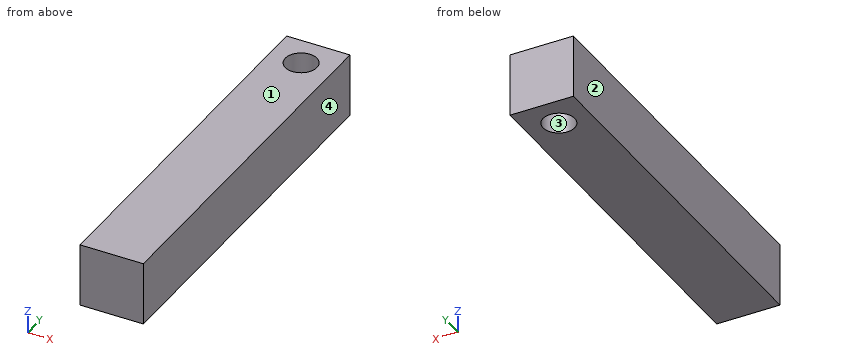
Autodesk Inventor part; units mm, degrees
ref_plane "YZ Plane" through (0, 0, 0) normal (1, 0, 0) x (0, 1, 0)
ref_plane "XZ Plane" through (0, 0, 0) normal (0, 1, 0) x (-1, 0, 0)
ref_plane "XY Plane" through (0, 0, 0) normal (0, 0, 1) x (1, 0, 0)
sketch "Sketch1" plane through (0, 0, 0) normal (0, 1, 0) x (-1, 0, 0)
  line L0 (0, 0) -> (-25.4, 0)
  line L1 (-25.4, 0) -> (-25.4, -25.4)
  line L2 (-25.4, -25.4) -> (0, -25.4)
  line L3 (0, -25.4) -> (0, 0)
  dimension "d0" = 25.4
  dimension "d1" = 25.4
extrude "Extrusion1" add sketch "Sketch1" along normal blind 152.4
sketch "Sketch2" plane through (25.4, 0, -25.4) normal (0, 0, -1) x (-1, 0, 0)
  circle A0 centre (12.7, 139.7) radius 6.35
  line L0 (0, 0) -> (0, 152.4)
  line L1 (0, 152.4) -> (25.4, 152.4)
  point P0 (25.4, 0)
  dimension "d4" = 12.7
  dimension "d5" = 12.7
  dimension "d6" = 12.7
extrude "Extrusion2" cut sketch "Sketch2" against normal blind 152.4
properties material "Aluminum 6061"
Can you work these out from the model? Positions are in its coordinate system, mm. Face numbers are marked on the shaded views. Give positions to 0.01 mm unless a question says otherwise; leave off trailing zeros. Loops run counter-clockwise (first coordinate to the right, second up) from the corner with the lowest first, then second, coordinate; pieces in that order, holes last. Notation, with made-up numbers: M 25.25,21.5 L 30.25,21.5 A12 cw 30.25,32.5 Z; hole C 18.5,86 d2. An arc over 180 degrees is marked long. Use one line per item in the form item = value. Start each with the question number.
(1) Thinking about a two-plate mould opening in X: for the marked faces 1, 2, 3 and 4, which applies, released by +X, released by -X, zero draft, split by the parting line, or undercut?
(2) I want a section at B-B, the plane y = 139.7. Write out the boundary of the cut face in (x, z), and give its area (3 significant figures).
(3) Please list where these lines run through material, in increasing order: line 1 (Y direction, x = 12.75, z = -14); line 2 (Y direction, x = 17.25, z = -15); line 3 (X direction, y = 135.5, z = -16).
(4) I want a section at C-C, the plane z = -19. Write out the boundary of the cut face in (x, y), and give its area (3 significant figures).
(5) I want a section at A-A, the plane x = 12.7. Write out the boundary of the cut face in (y, z), and give its area (3 significant figures).
Worked out:
q1.face_1 = zero draft
q1.face_2 = released by -X
q1.face_3 = undercut
q1.face_4 = released by +X
q2.outline = M 0,-25.4 L 6.35,-25.4 L 6.35,0 L 0,0 Z; M 19.05,-25.4 L 25.4,-25.4 L 25.4,0 L 19.05,0 Z
q2.area = 323 mm²
q3.line_1 = 0 to 133.35, 146.05 to 152.4
q3.line_2 = 0 to 135.27, 144.13 to 152.4
q3.line_3 = 0 to 7.94, 17.46 to 25.4
q4.outline = M 0,0 L 25.4,0 L 25.4,152.4 L 0,152.4 Z; hole C 12.7,139.7 d12.7
q4.area = 3,740 mm²
q5.outline = M 0,-25.4 L 133.35,-25.4 L 133.35,0 L 0,0 Z; M 146.05,-25.4 L 152.4,-25.4 L 152.4,0 L 146.05,0 Z
q5.area = 3,550 mm²
